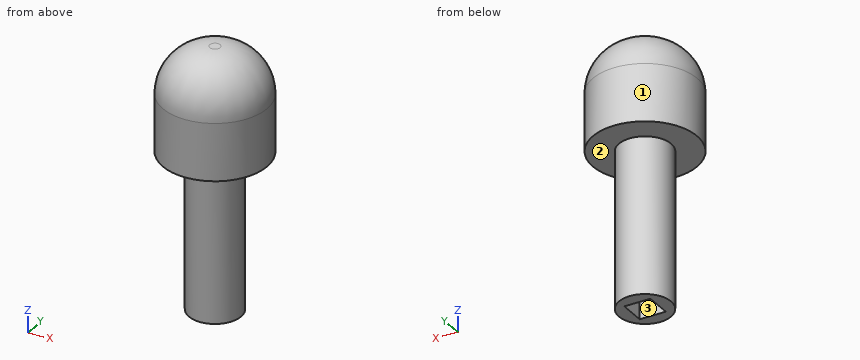
from build123d import *

# Parameters (mm, degrees)
SKETCH1_R           = 2
BASE_EXTRUDE_DEPTH  = 4
FILLET1_R           = 1.8
SKETCH2_R           = 1
BOSS_EXTRUDE1_DEPTH = 6
SKETCH3_W           = 1
SKETCH3_H           = 1
CUT_EXTRUDE1_DEPTH  = 1


with BuildPart() as part:
    # Sketch1 → Base-Extrude (new body)
    with BuildSketch(Plane.XY):
        Circle(SKETCH1_R)
    extrude(amount=-BASE_EXTRUDE_DEPTH)

    # Fillet1
    fillet1_edges = [part.edges().sort_by_distance(p)[0] for p in [
        (-2, 0, 0),
    ]]
    fillet(fillet1_edges, radius=FILLET1_R)

    # Sketch2 → Boss-Extrude1 (add)
    with BuildSketch(Plane(origin=(0, 0, -4), x_dir=(-1, 0, 0), z_dir=(0, 0, -1))):
        with Locations(Location((0, 0, 0), (0, 0, 180))):
            Circle(SKETCH2_R)
    extrude(amount=BOSS_EXTRUDE1_DEPTH)

    # Sketch3 → Cut-Extrude1 (cut)
    with BuildSketch(Plane(origin=(0, 0, -10), x_dir=(-1, 0, 0), z_dir=(0, 0, -1))):
        Rectangle(SKETCH3_W, SKETCH3_H)
    extrude(amount=-CUT_EXTRUDE1_DEPTH, mode=Mode.SUBTRACT)


solid = part.part
Can you work these out from the model? Positions are in its coordinate system, mm. Face numbers are marked on the shaded views. Give positions to 0.01 mm unless a question says otherwise; leave off trailing zeros. Write each loop counter-clockwise with the first axis right and the second up, starting at its lowest first coordinate (ties: lowest second). Pieces come first, ordered by that corner, then holes. Notation, with made-up numbers: M 24.25,1 L 49.25,1 A24 ccw 49.25,14 Z; hole C 73.25,-38.75 d10. An arc over 180 degrees is marked long. Answer in a Markdown table with one row per item. Add a question column.
Item 1: We'd pull the mould along X, two halves only. Please class the marked faces 1, 2 and 3: released by +X, released by -X, zero draft, split by the parting line, or undercut.
Item 2: For pin 1 Ø1.1 at (y, z) = (0, -9.5) entering from +X; pin 2 Ø0.8 at (x, z) = (0, -9.5) entering from -Y; pin 3 Ø0.8 at (x, y) = (0, 0) entering from -Z, each with a flat end and sliding along its axis, tell me the tip position at first contact or that it passes through.
Item 3: Please list where these lines run through material, in increasing order: L1, parallel to Z at x = 0, y = -0.1; L2, parallel to Y at x = 1.1, z = -2.75; L3, parallel to Z at x = -1.65, y = -0.35.
Item 4: Imagine slicing it at B-B, the plane z = -5.25. Write out the boundary of the cut face in (x, y), plus the area to 3 significant figures.
Item 5: Imagine slicing it at A-A, the plane z = -2.5. Write out the boundary of the cut face in (x, y), plus the area to 3 significant figures.
Evaluation:
| question | item | result |
|---|---|---|
| 1 | face 1 | split by the parting line |
| 1 | face 2 | zero draft |
| 1 | face 3 | undercut |
| 2 | pin 1 | stops at x = 1 |
| 2 | pin 2 | stops at y = -1 |
| 2 | pin 3 | stops at z = -9 |
| 3 | L1 | z = -9 to 0 |
| 3 | L2 | y = -1.67 to 1.67 |
| 3 | L3 | z = -4 to -0.79 |
| 4 | outline | C 0,0 d2 |
| 4 | area | 3.14 mm² |
| 5 | outline | C 0,0 d4 |
| 5 | area | 12.6 mm² |
